Could you check a few things on this model? Use its own coordinates, in mm. Round coordinates to 2 decimals unless told otherwise and drop trailing zeros. Write each loop counter-clockwise with the first axis right and the second up, starting at its lowest first coordinate (ties: lowest second). Pieces come first, ordered by that corner, then holes.
Autodesk Inventor part; units mm, degrees
ref_plane "YZ Plane" through (0, 0, 0) normal (1, 0, 0) x (0, 1, 0)
ref_plane "XZ Plane" through (0, 0, 0) normal (0, 1, 0) x (-1, 0, 0)
ref_plane "XY Plane" through (0, 0, 0) normal (0, 0, 1) x (1, 0, 0)
sketch "Sketch12" plane through (0, 0, 0) normal (0, 0, 1) x (1, 0, 0)
  line L0 (0, 0) -> (35, 0)
  line L1 (35, 0) -> (35, 47)
  line L2 (35, 47) -> (0, 47)
  line L3 (0, 47) -> (0, 0)
  line L4 (0, 47) -> (2, 47) construction
  line L5 (2, 47) -> (2, 35.5) construction
  line L6 (35, 47) -> (33, 47) construction
  line L7 (33, 47) -> (33, 35.5) construction
  circle A0 centre (33, 35.5) radius 1.25
  circle A1 centre (2, 35.5) radius 1.25
  line L8 (0, 0) -> (6.5, 0) construction
  line L9 (35, 0) -> (28.5, 0) construction
  line L10 (6.5, 0) -> (6.5, 3.2) construction
  line L11 (28.5, 0) -> (28.5, 3.2) construction
  circle A2 centre (6.5, 3.2) radius 1.25
  circle A3 centre (28.5, 3.2) radius 1.25
  dimension "d49" = 35
  dimension "d50" = 47
  dimension "d97" = 2
  dimension "d98" = 11.5
  dimension "d99" = 2
  dimension "d100" = 2.5
  dimension "d101" = 2.5
  dimension "d102" = 11.5
  dimension "d103" = 6.5
  dimension "d104" = 6.5
  dimension "d105" = 3.2
  dimension "d106" = 3.2
  dimension "d107" = 2.5
  dimension "d108" = 2.5
extrude "Extrusión8" add sketch "Sketch12" along normal blind 4
sketch "Boceto21" plane through (0, 0, 0) normal (0, -1, 0) x (1, 0, 0)
  line L0 (35, 0) -> (35, 4) construction
  line L1 (35, 0) -> (35, 4) construction
  line L2 (0, 0) -> (0, 4) construction
  line L3 (0, 0) -> (0, 4) construction
  line L4 (0, 2) -> (35, 2) construction
  line L5 (35, 2) -> (25, 2) construction
  line L6 (0, 2) -> (9, 2) construction
  circle A0 centre (9, 2) radius 1.5
  circle A1 centre (25, 2) radius 1.5
  dimension "d111" = 10
  dimension "d112" = 9
  dimension "d113" = 3
  dimension "d114" = 3
extrude "Extrusión9" cut sketch "Boceto21" along normal through all both and the other way through all
equation "\"BendRadius\" = Thickness"
equation "\"BendReliefWidth\" = Thickness"
equation "\"BendReliefDepth\" = 0.5 * Thickness"
equation "\"CornerReliefSize\" = 4 * Thickness"
equation "\"MinimumRemnant\" = 2 * Thickness"
equation "\"TransitionRadius\" = BendRadius"
equation "\"JacobiRadiusSize\" = BendRadius"
equation "\"GapSize\" = Thickness"
properties part number "Suportmotor"
Q1. Imagine slicing it at A-A, the plane z = 2. Write out the boundary of the cut face in (x, y).
Q2. We'd pull the mould along X, two halves only. Please class faces 1 (the cylindrical face through (5.25, 3.15, 1.97)), 2 (the flat face through (35, 23, 2)), 3 (the flat face through (0, 24, 2)): pulls with the +X half, pulls with the -X half, needs draft (parallel to the pull), parting line crosses it, or undercut.
Q3. Imagine slicing it at C-C, the plane x = 6.5. Write out the boundary of the cut face in (y, z), then the cut area to 3 significant figures.
Q4. Imagine slicing it at B-B, the plane y = 35.5. Write out the boundary of the cut face in (x, z).
Q5. Imagine slicing it at D-D, the plane y = 3.2. Write out the boundary of the cut face in (x, z), then the cut area to 3 significant figures.
Q6. If I drill on L1, parallel to X at y = 38.5, z = 2.1; L2, parallel to Z at x = 25, y = 17.5; L3, parallel to X at y = 30, z = 1.3, over which ranges is the centre line in solid material (lowest first)?
Results found:
1. outline: (0, 0) - (7.5, 0) - (7.5, 2.45) arc R1.25 cw (long way) to (7.5, 3.95) - (7.5, 47) - (0, 47) - close; (10.5, 0) - (23.5, 0) - (23.5, 47) - (10.5, 47) - close; (26.5, 0) - (35, 0) - (35, 47) - (26.5, 47) - close; hole circle Ø2.5 at (2, 35.5); hole circle Ø2.5 at (28.5, 3.2); hole circle Ø2.5 at (33, 35.5)
2. face 1: undercut
2. face 2: pulls with the +X half
2. face 3: pulls with the -X half
3. outline: (0, 0) - (1.95, 0) - (1.95, 4) - (0, 4) - close; (4.45, 0) - (47, 0) - (47, 4) - (4.45, 4) - close
3. area: 178 mm2
4. outline: (0, 0) - (0.75, 0) - (0.75, 4) - (0, 4) - close; (3.25, 0) - (31.75, 0) - (31.75, 4) - (3.25, 4) - close; (34.25, 0) - (35, 0) - (35, 4) - (34.25, 4) - close; hole circle Ø3 at (9, 2); hole circle Ø3 at (25, 2)
5. outline: (0, 0) - (5.25, 0) - (5.25, 4) - (0, 4) - close; (7.75, 0) - (27.25, 0) - (27.25, 4) - (7.75, 4) - (7.75, 2.83) arc R1.5 cw (long way) to (7.75, 1.17) - close; (29.75, 0) - (35, 0) - (35, 4) - (29.75, 4) - close; hole circle Ø3 at (25, 2)
5. area: 106 mm2
6. L1: x = 0 to 7.5, 10.5 to 23.5, 26.5 to 35
6. L2: z = 0 to 0.5, 3.5 to 4
6. L3: x = 0 to 7.67, 10.33 to 23.67, 26.33 to 35
